Read the model definition and answer for the solid it produces. Units are mm, in the model's axes. Round coordinates to 2 decimals unless told otherwise and drop trailing zeros. Loops run counter-clockwise (first coordinate to the right, second up) from the corner with the lowest first, then second, coordinate; pieces in that order, holes last. Notation, with made-up numbers: M 77.25,68.25 L 95.25,68.25 A28 cw 95.25,105.25 Z; hole C 73,-3.75 d6. An arc over 180 degrees is marked long. Write each question's results on one line, items separated by ' | '.
from build123d import *

# Parameters (mm, degrees)
BOSS_EXTRUDE1_DEPTH                                = 6.35
SKETCH2_W                                          = 33.274
SKETCH2_H                                          = 381
CUT_EXTRUDE1_DEPTH                                 = 7.35
CSK_FOR_10_FLAT_HEAD_MACHINE_SCREW_100_D           = 5.1054
CSK_FOR_10_FLAT_HEAD_MACHINE_SCREW_100_CSINK_D     = 9.779
CSK_FOR_10_FLAT_HEAD_MACHINE_SCREW_100_CSINK_ANGLE = 100


with BuildPart() as part:
    # Sketch1 → Boss-Extrude1 (new body)
    with BuildSketch(Plane.XY):
        with BuildLine():
            Line((141.422179454, -15.387658672), (141.422179454, -76.238562419))
            Line((141.422179454, -76.238562419), (133.548179454, -76.238562419))
            Line((133.548179454, -76.238562419), (-101.401820546, -76.238562419))
            Line((-101.401820546, -76.238562419), (-101.401820546, 304.761437581))
            Line((-101.401820546, 304.761437581), (0, 304.761437581))
            Line((0, 304.761437581), (20.828, 304.761437581))
            Line((20.828, 304.761437581), (20.828, 110.451437581))
            ThreePointArc((20.828, 110.451437581), (21.317531228, 108.006564216), (22.710647487, 105.938648918))
            Line((22.710647487, 105.938648918), (139.539531967, -10.874870008))
            ThreePointArc((139.539531967, -10.874870008), (140.932648226, -12.942785307), (141.422179454, -15.387658672))
        make_face()
    extrude(amount=BOSS_EXTRUDE1_DEPTH)

    # Sketch2 → Cut-Extrude1 (cut, through all)
    with BuildSketch(Plane.XY.offset(6.35)):
        with Locations((-84.764820546, 114.261437581)):
            Rectangle(SKETCH2_W, SKETCH2_H)
    extrude(amount=-CUT_EXTRUDE1_DEPTH, mode=Mode.SUBTRACT)

    # CSK for #10 Flat Head Machine Screw (100)1 (through all)
    with Locations(Plane(origin=(119.832179454, -0.038562419, 0), x_dir=(-1, 0, 0), z_dir=(0, 0, -1))):
        with Locations((0, 0), (89.916, 89.916), (105.41, 139.7), (105.41, 266.7)):
            CounterSinkHole(CSK_FOR_10_FLAT_HEAD_MACHINE_SCREW_100_D / 2, CSK_FOR_10_FLAT_HEAD_MACHINE_SCREW_100_CSINK_D / 2, counter_sink_angle=CSK_FOR_10_FLAT_HEAD_MACHINE_SCREW_100_CSINK_ANGLE)


solid = part.part
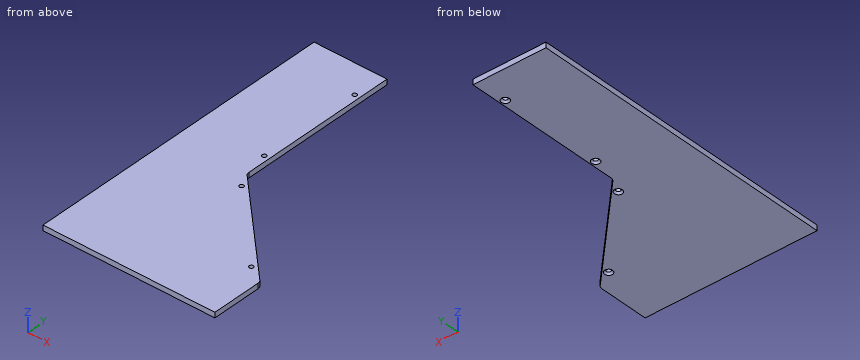
Item 1: The part is cut by section B-B (y = 22). Determine the outline of the cut face in (x, z).
Outcome:
outline: M -68.13,0 L 106.66,0 L 106.66,6.35 L -68.13,6.35 Z
Item 2: The part is cut by section A-A (z = 4.5). Determine the outline of the cut face in (x, y), plus the area to 3 significant figures.
Outcome:
outline: M -68.13,-76.24 L 141.42,-76.24 L 141.42,-15.39 A6.35 ccw 139.54,-10.87 L 22.71,105.94 A6.35 cw 20.83,110.45 L 20.83,304.76 L -68.13,304.76 Z; hole C 14.42,139.66 d5.11; hole C 14.42,266.66 d5.11; hole C 29.92,89.88 d5.11; hole C 119.83,-0.04 d5.11 | area: 48,700 mm2
Item 3: The part is cut by section C-C (x = 67). Determine the outline of the cut face in (y, z), plus the area to 3 significant figures.
Outcome:
outline: M -76.24,0 L 61.66,0 L 61.66,6.35 L -76.24,6.35 Z | area: 876 mm2
Item 4: Flat-ended cylindrical pins translate along their axes: pin 1 (8 mm diameter, centred on x = 14.42, y = 139.66, fed in from -Z); pin 2 (1.9 mm diameter, centred on y = 166.5, z = 4.5, fed in from +X). Find the tip coordinate at first contact, or state that the pin passes through.
Outcome:
pin 1: stops at z = 0.74 | pin 2: stops at x = 20.83
Item 5: Straight lines are drawn through the part: line 1 (X direction, y = 158, z = 5.75); line 2 (Y direction, x = 52.5, z = 4.5); line 3 (X direction, y = 14.5, z = 2.5). For each, find the intervals that lie inside material, in ascending order.
Outcome:
line 1: x = -68.13 to 20.83 | line 2: y = -76.24 to 76.15 | line 3: x = -68.13 to 114.16
